from build123d import *

# Parameters (mm, degrees)
SKETCH_1_W               = 41.11
SKETCH_1_H               = 18.14
SKETCH_1_R               = 5.25
EXTRUDE_1_DEPTH          = 3.5
SKETCH_3_W               = 3.5
SKETCH_3_H               = 18.14
EXTRUDE_2_DEPTH          = 7
CUT_EXTRUDE_1_DEPTH      = 45.116640965
CUT_EXTRUDE_1_DEPTH_BACK = 45.116640965
SKETCH_4_R               = 1.5
FILLET_1_R               = 1
FILLET_2_R               = 3


with BuildPart() as part:
    # 草图1 → 凸台-拉伸1 (new body)
    with BuildSketch(Plane.XY):
        with Locations((-11.958959751, -3.012876727)):
            Rectangle(SKETCH_1_W, SKETCH_1_H)
        with Locations((-17.483959751, -3.012876727)):
            Circle(SKETCH_1_R, mode=Mode.SUBTRACT)
    extrude(amount=EXTRUDE_1_DEPTH)

    # 草图3 → 凸台-拉伸2 (add)
    with BuildSketch(Plane.XY.offset(3.5)):
        with Locations((-30.763959751, -3.012876727)):
            Rectangle(SKETCH_3_W, SKETCH_3_H)
        with Locations((6.846040249, -3.012876727)):
            Rectangle(SKETCH_3_W, SKETCH_3_H)
    extrude(amount=EXTRUDE_2_DEPTH)

    # 草图4 → 切除-拉伸1 (cut, two sides: drawn at the far end of the back side and taken through both)
    with BuildSketch(Plane(origin=(8.596040249, 0, 0), x_dir=(0, 0, -1), z_dir=(1, 0, 0)).offset(-CUT_EXTRUDE_1_DEPTH_BACK)):
        with Locations(Location((-7.5, 1.987123273, 0), (0, 0, 90))):
            Circle(SKETCH_4_R)
        with Locations(Location((-7.5, -8.012876727, 0), (0, 0, 90))):
            Circle(SKETCH_4_R)
    extrude(amount=CUT_EXTRUDE_1_DEPTH + CUT_EXTRUDE_1_DEPTH_BACK, mode=Mode.SUBTRACT)

    # 圆角1
    fillet_1_edges = [part.edges().sort_by_distance(p)[0] for p in [
        (-29.013959751, -3.012876727, 3.5),
        (5.096040249, -3.012876727, 3.5),
    ]]
    fillet(fillet_1_edges, radius=FILLET_1_R)

    # 圆角2
    fillet_2_edges = [part.edges().sort_by_distance(p)[0] for p in [
        (-30.763959751, -12.082876727, 10.5),
        (-30.763959751, 6.057123273, 10.5),
        (6.846040249, 6.057123273, 10.5),
        (6.846040249, -12.082876727, 10.5),
    ]]
    fillet(fillet_2_edges, radius=FILLET_2_R)


solid = part.part
Input: part model. Units: mm. Frame: model coordinates. A direction names the side the tool comes from. Round coordinates to 2 decimals unless told otherwise and drop trailing zeros. Order: outer loops, then holes, each group sorted by start corner. A loop starts at its lowest first (then second) coordinate and runs counter-clockwise, first axis right, second up. Notation, with made-up numbers: (-2, 65) - (19, 65) arc R31 cw to (19, 102) - close; hole circle Ø9 at (10, 89.25). An arc over 180 degrees is marked (long way). Answer as a JSON object with one key per item and string values. Group by question number.
(1) Material intervals for probe 1 along Y at (x, z) = (7.9, 7.5); probe 2 along X at (y, z) = (-6.5, 9.75); probe 3 along Z at (x, y) = (-4, -0.5), sorted ascending. Write a range as from..to.
(2) Cut plane A-A (x = 5.5). Return loops of the section in (y, z), then the cut area to 3 significant figures.
(3) Draft query along X for faces 1 (the face through (4.8, -2.89, 3.79)), 2 (the face through (-12, -12.083, 2)), 3 (the face through (8.596, -3, 5)), 4 (the face through (-12, -3, 3.5)). Return one class per face: released by +X, released by -X, zero draft, split by the parting line, or undercut.
(4) Cut plane C-C (z = 2). Return loops of the section in (x, y), then the cut area to 3 significant figures.
(5) Pin query (flat end, axial travel): P1, Ø2.5, axis at y = -8.01, z = 7.5, coming from the +X side; P2, Ø9, axis at x = -7, y = -3.5, coming from the +Z side. Return the tip coordinate at first contact, or that it passes through.
(6) Cut plane B-B (y = 1). Return loops of the section in (x, z).
(7) Reachability of faces 5 (the face through (5.096, -3, 7)), 6 (the face through (-32.514, -3, 5)) from +Z, -Z, +X, -X, +Y, -Y: full face, straight path, thin tool, end or side. Return the list, or none.
(8) Cut plane D-D (y = -3.75). Return loops of the section in (x, z), then the cut area to 3 significant figures.
Here are the results:
{
 "1": {"probe 1": "y = -12.08..-9.51, -6.51..0.49, 3.49..6.06", "probe 2": "x = -32.51..-29.01, 5.1..8.6", "probe 3": "z = 0..3.5"},
 "2": {"outline": "(-12.08, 0) - (6.06, 0) - (6.06, 7.5) arc R3 ccw to (3.06, 10.5) - (-9.08, 10.5) arc R3 ccw to (-12.08, 7.5) - close; hole circle Ø3 at (-8.01, 7.5); hole circle Ø3 at (1.99, 7.5)", "area": "172 mm^2"},
 "3": {"face 1": "undercut", "face 2": "zero draft", "face 3": "released by +X", "face 4": "undercut"},
 "4": {"outline": "(-32.51, -12.08) - (8.6, -12.08) - (8.6, 6.06) - (-32.51, 6.06) - close; hole circle Ø10.5 at (-17.48, -3.01)", "area": "659 mm^2"},
 "5": {"P1": "passes through", "P2": "stops at z = 3.5"},
 "6": {"outline": "(-32.51, 0) - (-20.87, 0) - (-20.87, 3.5) - (-28.01, 3.5) arc R1 cw to (-29.01, 4.5) - (-29.01, 6.37) - (-32.51, 6.37) - close; (-32.51, 8.63) - (-29.01, 8.63) - (-29.01, 10.5) - (-32.51, 10.5) - close; (-14.1, 0) - (8.6, 0) - (8.6, 6.37) - (5.1, 6.37) - (5.1, 4.5) arc R1 cw to (4.1, 3.5) - (-14.1, 3.5) - close; (5.1, 8.63) - (8.6, 8.63) - (8.6, 10.5) - (5.1, 10.5) - close"},
 "7": {"face 5": "+Z, +Y, -Y", "face 6": "+Z, -Z, -X, +Y, -Y"},
 "8": {"outline": "(-32.51, 0) - (-22.68, 0) - (-22.68, 3.5) - (-28.01, 3.5) arc R1 cw to (-29.01, 4.5) - (-29.01, 10.5) - (-32.51, 10.5) - close; (-12.29, 0) - (8.6, 0) - (8.6, 10.5) - (5.1, 10.5) - (5.1, 4.5) arc R1 cw to (4.1, 3.5) - (-12.29, 3.5) - close", "area": "157 mm^2"}
}
